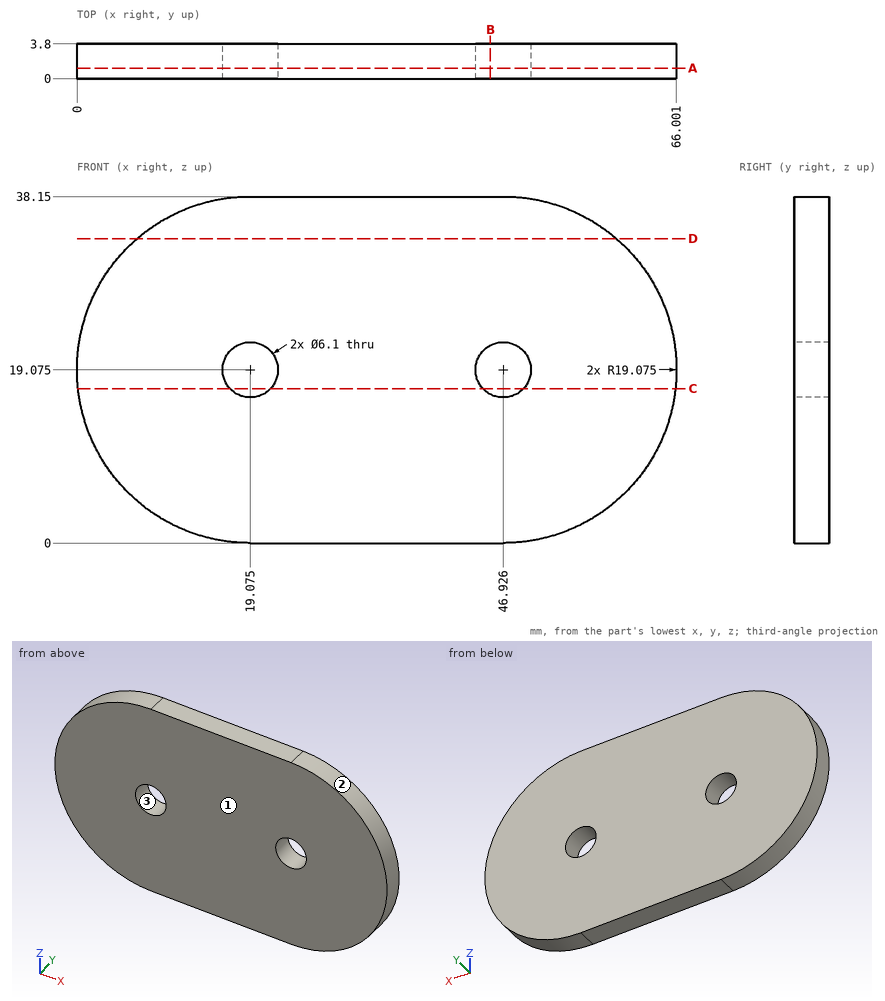
Study the drawing (mm; zero at the part's minimum x, y, z) and answer. Round coordinates to 2 decimals unless told otherwise and drop trailing zeros. Order: outer loops, then holes, each group sorted by start corner. A loop starts at its lowest first (then second) coordinate and runs counter-clockwise, first axis right, second up. Notation, with made-up numbers: (-2.5, -9.5) -> (1.5, -9.5) arc R24 cw to (1.5, 9.5) -> close; hole circle Ø9 at (30.25, 51). An arc over 180 degrees is marked (long way). Answer as CSV lines item,"result". Start each with the question number.
(1) Flat-ended cylindrical pins translate along their axes: pin 1 Ø1 at (x, y) = (52.5, 2) entering from -Z; pin 2 Ø1.5 at (x, y) = (50.5, 0.5) entering from +Z. Find the tip coordinate at first contact, or state that the pin passes through.
(2) The part is cut by section D-D (z = 33.5). Determine the outline of the cut face in (x, y), then the cut area to 3 significant figures.
(3) The part is cut by section B-B (x = 45.5). Determine the outline of the cut face in (y, z).
(4) For a pull along Z with two mould halves and no side action, classify the marked faces 1, 2 and 3 as +Z half, -Z half, draft (parallel to the pull), parting line (faces both ways), or undercut.
(5) Find the intervals of material crossed by probe 1 along X at (y, z) = (1.75, 20.5); probe 2 along Z at (x, y) = (20, 3.55); probe 3 along Z at (x, y) = (16.5, 0.7) (1 decimal), in increasing order. Write a range as from..to.
(6) The part is cut by section A-A (y = 1.15). Count the separate pieces of the cut face and the enclosed holes in it, then the cut area to 3 significant figures.
(7) The part is cut by section C-C (z = 17). Determine the outline of the cut face in (x, y).
Evaluation:
1,pin 1,"z = 0.69"
1,pin 2,"z = 37.94"
2,outline,"(6.59, 0) -> (59.41, 0) -> (59.41, 3.8) -> (6.59, 3.8) -> close"
2,area,"201 mm²"
3,outline,"(0, 0) -> (3.8, 0) -> (3.8, 16.38) -> (0, 16.38) -> close; (0, 21.77) -> (3.8, 21.77) -> (3.8, 38.15) -> (0, 38.15) -> close"
4,face 1,"draft"
4,face 2,"parting line"
4,face 3,"undercut"
5,probe 1,"0.05..16.38, 21.77..44.23, 49.62..65.95"
5,probe 2,"0..16.17, 21.98..38.15"
5,probe 3,"0.2..17.4, 20.7..38"
6,separate pieces,"1"
6,enclosed holes,"2"
6,area,"2,150 mm²"
7,outline,"(0.11, 0) -> (16.84, 0) -> (16.84, 3.8) -> (0.11, 3.8) -> close; (21.31, 0) -> (44.69, 0) -> (44.69, 3.8) -> (21.31, 3.8) -> close; (49.16, 0) -> (65.89, 0) -> (65.89, 3.8) -> (49.16, 3.8) -> close"
